Autodesk Inventor part; units mm, degrees
ref_plane "YZ Plane" through (0, 0, 0) normal (1, 0, 0) x (0, 1, 0)
ref_plane "XZ Plane" through (0, 0, 0) normal (0, 1, 0) x (-1, 0, 0)
ref_plane "XY Plane" through (0, 0, 0) normal (0, 0, 1) x (1, 0, 0)
sketch "Sketch1" plane through (0, 0, 0) normal (0, 1, 0) x (-1, 0, 0)
  line L0 (0, 0) -> (0, -164)
  line L1 (0, 0) -> (-9, 0)
  line L2 (0, -164) -> (-9, -164)
  line L3 (56.0828, -82) -> (-131.3763, -82) construction
  arc A0 (-146.3035, -74.0793) -> (-146.3035, -89.9207) centre (-142.03, -82) ccw
  line L4 (-110.9841, -85.4733) -> (-28.9841, -132.315)
  line L5 (-110.9833, -78.5263) -> (-28.9833, -31.7073)
  arc A1 (-23, -35.1809) -> (-28.9833, -31.7073) centre (-27, -35.1809) ccw
  arc A2 (-28.9841, -132.315) -> (-23, -128.8417) centre (-27, -128.8417) ccw
  line L6 (-23, -35.1809) -> (-23, -128.8417)
  line L7 (-146.3035, -89.9207) -> (-9, -164)
  line L8 (-9, 0) -> (-146.3035, -74.0793)
  arc A3 (-110.9833, -78.5263) -> (-110.9841, -85.4733) centre (-109, -82) ccw
  point P0 (0, -82)
  point P1 (-23, -82)
  point P2 (-75.5556, -35.9087)
  point P3 (-69.9833, -55.1168)
  point P4 (-75.5113, -128.1152)
  point P5 (-69.9841, -108.8941)
  dimension "d0" = 164
  dimension "d1" = 9
  dimension "d2" = 9
  dimension "d13" = 18
  dimension "d20" = 8
  dimension "d21" = 8
  dimension "d73" = 142.03
  dimension "d74" = 23
  dimension "d76" = 8
  dimension "d77" = 86
  dimension "d78" = 20
  dimension "d79" = 20
extrude "Extrusion1" add sketch "Sketch1" along normal blind 5
sketch "Sketch2" plane through (0, 5, 0) normal (0, 1, 0) x (1, 0, 0)
  line L0 (0, 164) -> (0, 0)
  line L1 (0, 82) -> (160.3523, 82) construction
  line L2 (4.5, 12) -> (4.5, 152) construction
  circle A0 centre (4.5, 12) radius 2
  circle A1 centre (4.5, 152) radius 2
  line L3 (23, 12.6666) -> (23, 144.7978) construction
  circle A2 centre (23, 12.6666) radius 2
  line L4 (23, 12.6666) -> (151.5071, 82) construction
  circle A3 centre (54.2428, 29.523) radius 2
  circle A4 centre (69.8202, 37.9275) radius 2
  line L5 (9, 0) -> (146.3035, 74.0793)
  circle A5 centre (85.3976, 46.3319) radius 2
  circle A6 centre (100.9749, 54.7364) radius 2
  circle A7 centre (116.5523, 63.1409) radius 2
  circle A8 centre (132.1297, 71.5453) radius 2
  circle A9 centre (38.6654, 21.1185) radius 2
  circle A10 centre (23, 151.3334) radius 2
  circle A11 centre (54.2428, 134.477) radius 2
  circle A12 centre (69.8202, 126.0725) radius 2
  circle A13 centre (85.3976, 117.6681) radius 2
  circle A14 centre (116.5523, 100.8591) radius 2
  circle A15 centre (132.1297, 92.4547) radius 2
  circle A16 centre (38.6654, 142.8815) radius 2
  point P0 (4.5, 82)
  point P1 (100.9749, 109.2636)
  dimension "d82" = 4
  dimension "d83" = 4
  dimension "d84" = 140
  dimension "d85" = 4.5
  dimension "d88" = 4
  dimension "d89" = 4
  dimension "d91" = 4
  dimension "d93" = 23
  dimension "d94" = 4.5
  dimension "d95" = 4.5
  dimension "d98" = 4
  dimension "d99" = 4
  dimension "d100" = 4
  dimension "d101" = 4
  dimension "d106" = 17.7
  dimension "d107" = 17.7
  dimension "d108" = 17.7
  dimension "d109" = 17.7
  dimension "d110" = 124
  dimension "d111" = 17.7
  dimension "d112" = 4
  dimension "d113" = 17.7
hole "Hole2" at (4.5, 5, -12) at (23, 5, -12.6666) at (4.5, 5, -152) at (23, 5, -151.3334) direction (0, -1, 0) diameter 4 depth 10 tip angle 118
equation "\"d95\" = d94"
properties part number "17 nueva"
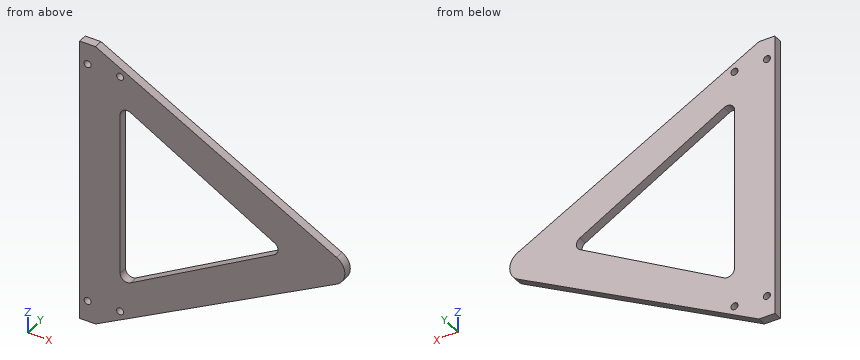
The model under review builds one solid part; all positions refer to its coordinate system, in mm. Round coordinates to 2 decimals unless told otherwise and drop trailing zeros. Order: outer loops, then holes, each group sorted by start corner. A loop starts at its lowest first (then second) coordinate and runs counter-clockwise, first axis right, second up. Notation, with made-up numbers: (58, 31.25) - (75, 31.25) arc R30 ccw to (75, 53.25) - close; hole circle Ø4 at (-20, -4). An arc over 180 degrees is marked (long way). Use one line per item in the form item = value.
Q1. Add section C-C on z = -92. Give the boundary of the cut face in (x, y), then the cut area to 3 significant figures.
Response values:
outline = (0, 0) - (23, 0) - (23, 5) - (0, 5) - close; (99.56, 0) - (142.45, 0) - (142.45, 5) - (99.56, 5) - close
area = 329 mm^2
Q2. To check wall thickness, follow line 1 (X direction, y = 3.45, z = -152); line 2 (Z direction, x = 101.5, y = 3.5); line 3 (X direction, y = 2.6, z = -93.5). State the ranges of each line that lie inside material, in increasing order.
Response values:
line_1 = 0 to 2.5, 6.5 to 21.11, 24.89 to 31.24
line_2 = -114.09 to -90.89, -73.11 to -49.91
line_3 = 0 to 23, 96.93 to 139.67
Q3. Clearance check with flat-ended pins moving along their axes: P1, Ø3, axis at x = 28, y = 3.5, coming from the -Z side; P2, Ø2.5, axis at x = 23, z = -151.33, coming from the +Y side; P3, Ø2.5, axis at y = 2.5, z = -104, coming from the +X side; P4, Ø3, axis at x = 103.5, y = 2, coming from the +Z side. State where each tip first meets the part, or that it passes through.
Response values:
P1 = -154.56
P2 = through
P3 = 122.52
P4 = -50.18
Q4. Add section B-B on x = 4.5. Give the boundary of the cut face in (y, z), then the cut area to 3 significant figures.
Response values:
outline = (0, -164) - (5, -164) - (5, -154) - (0, -154) - close; (0, -150) - (5, -150) - (5, -14) - (0, -14) - close; (0, -10) - (5, -10) - (5, 0) - (0, 0) - close
area = 780 mm^2
Q5. Add section D-D on x = 82. Give the boundary of the cut face in (y, z), then the cut area to 3 significant figures.
Response values:
outline = (0, -124.61) - (5, -124.61) - (5, -102.03) - (0, -102.03) - close; (0, -61.98) - (5, -61.98) - (5, -39.39) - (0, -39.39) - close
area = 226 mm^2
Q6. Add section A-A on y = 3.05. Give the boundary of the cut face in (x, z) (1 decimal).
Response values:
outline = (0, -164) - (9, -164) - (146.3, -89.9) arc R9 ccw to (146.3, -74.1) - (9, 0) - (0, 0) - close; hole circle Ø4 at (4.5, -152); hole circle Ø4 at (4.5, -12); hole circle Ø4 at (23, -151.3); hole circle Ø4 at (23, -12.7); hole (23, -128.8) arc R4 ccw to (29, -132.3) - (111, -85.5) arc R4 ccw to (111, -78.5) - (29, -31.7) arc R4 ccw to (23, -35.2) - close
